from build123d import *

# Parameters (mm, degrees)
SKETCH2_W           = 60
SKETCH2_H           = 10
SKETCH2_W_2         = 11.850089675
SKETCH2_H_2         = 89.916
SKETCH2_R           = 4
SKETCH2_W_3         = 10.16
SKETCH2_H_3         = 76.2
SKETCH2_R_2         = 3.175
SKETCH2_R_3         = 4.7625
SKETCH2_H_4         = 63.685061478
SKETCH2_H_5         = 63.685061479
BOSS_EXTRUDE1_DEPTH = 10


with BuildPart() as part:
    # Sketch2 → Boss-Extrude1 (new body)
    with BuildSketch(Plane.XY):
        with BuildLine():
            Line((-102.394461083, 316.728644457), (-121.859662508, 219.58578935))
            Line((-121.859662508, 219.58578935), (-459.721789204, 219.58578935))
            Line((-459.721789204, 219.58578935), (-459.721789204, -230.782639429))
            ThreePointArc((-459.721789204, -230.782639429), (-437.403325931, -284.664176156), (-383.521789204, -306.982639429))
            Line((-383.521789204, -306.982639429), (-252, -306.982639429))
            Line((-252, -306.982639429), (-252, -317.142639429))
            Line((-252, -317.142639429), (-55.8292, -317.142639429))
            Line((-55.8292, -317.142639429), (-55.8292, -306.982639429))
            Line((-55.8292, -306.982639429), (55.8292, -306.982639429))
            Line((55.8292, -306.982639429), (55.8292, -317.142639429))
            Line((55.8292, -317.142639429), (252, -317.142639429))
            Line((252, -317.142639429), (252, -306.982639429))
            Line((252, -306.982639429), (383.521789204, -306.982639429))
            ThreePointArc((383.521789204, -306.982639429), (437.403325931, -284.664176156), (459.721789204, -230.782639429))
            Line((459.721789204, -230.782639429), (459.721789204, 152.75736057))
            Line((459.721789204, 152.75736057), (408.921789204, 152.75736057))
            Line((408.921789204, 152.75736057), (411.84465756, 142.597360571))
            Line((411.84465756, 142.597360571), (335.64465756, 142.597360571))
            Line((335.64465756, 142.597360571), (335.022501884, 152.75736057))
            Line((335.022501884, 152.75736057), (135.250547773, 152.75736057))
            Line((135.250547773, 152.75736057), (102.394461083, 316.728644457))
            Line((102.394461083, 316.728644457), (-102.394461083, 316.728644457))
        make_face()
        with Locations((-365.16, -186.254154613)):
            Rectangle(SKETCH2_W, SKETCH2_H, mode=Mode.SUBTRACT)
        with Locations((-311.557332494, -172.10863943)):
            Rectangle(SKETCH2_W_2, SKETCH2_H_2, mode=Mode.SUBTRACT)
        with Locations((-240.16, -186.254154613)):
            Rectangle(SKETCH2_W, SKETCH2_H, mode=Mode.SUBTRACT)
        with Locations((-172.69, -269.442639429)):
            Circle(SKETCH2_R, mode=Mode.SUBTRACT)
        with Locations((-205.08, -256.782661115)):
            Rectangle(SKETCH2_W_3, SKETCH2_H_3, mode=Mode.SUBTRACT)
        with Locations((-172.69, -239.442639429)):
            Circle(SKETCH2_R, mode=Mode.SUBTRACT)
        with Locations((-117.38, -269.442639429)):
            Circle(SKETCH2_R, mode=Mode.SUBTRACT)
        with Locations((-117.38, -239.442639429)):
            Circle(SKETCH2_R, mode=Mode.SUBTRACT)
        with Locations((-84.92, -256.782661115)):
            Rectangle(SKETCH2_W_3, SKETCH2_H_3, mode=Mode.SUBTRACT)
        with BuildLine():
            ThreePointArc((-108.5, -194.170881029), (-95, -207.670881029), (-108.5, -221.170881029))
            Line((-108.5, -221.170881029), (-138.5, -221.170881029))
            ThreePointArc((-138.5, -221.170881029), (-152, -207.670881029), (-138.5, -194.170881029))
            Line((-138.5, -194.170881029), (-108.5, -194.170881029))
        make_face(mode=Mode.SUBTRACT)
        with Locations((-336.55027219, -94.687385458)):
            Circle(SKETCH2_R_2, mode=Mode.SUBTRACT)
        with Locations((-378.573819589, -5.78737531)):
            Circle(SKETCH2_R_2, mode=Mode.SUBTRACT)
        with Locations((-365.16, -74.446988355)):
            Rectangle(SKETCH2_W, SKETCH2_H, mode=Mode.SUBTRACT)
        Polygon((-270.16, -69.446988355), (-210.16, -69.446988355), (-210.16, -8.96237531), (-200, -8.96237531), (-200, -85.16237531), (-210.16, -85.16237531), (-210.16, -79.446988355), (-270.16, -79.446988355), align=None, mode=Mode.SUBTRACT)
        with Locations((-336.55027219, -5.787385458)):
            Circle(SKETCH2_R_2, mode=Mode.SUBTRACT)
        with Locations((-84.92, -47.06237531)):
            Rectangle(SKETCH2_W_3, SKETCH2_H_3, mode=Mode.SUBTRACT)
        with Locations((0, -78.38263943)):
            Circle(SKETCH2_R_2, mode=Mode.SUBTRACT)
        with Locations((311.557332494, -172.10863943)):
            Rectangle(SKETCH2_W_2, SKETCH2_H_2, mode=Mode.SUBTRACT)
        with Locations((95.25, -84.73263943)):
            Circle(SKETCH2_R_3, mode=Mode.SUBTRACT)
        with Locations((195.58, -147.752560311)):
            Rectangle(SKETCH2_W_3, SKETCH2_H_4, mode=Mode.SUBTRACT)
        with Locations((195.58, -20.382437355)):
            Rectangle(SKETCH2_W_3, SKETCH2_H_5, mode=Mode.SUBTRACT)
        with Locations((336.550272189, -94.687385458)):
            Circle(SKETCH2_R_2, mode=Mode.SUBTRACT)
        with Locations((336.550272189, -5.787385458)):
            Circle(SKETCH2_R_2, mode=Mode.SUBTRACT)
        with Locations((378.573819589, -5.78737531)):
            Circle(SKETCH2_R_2, mode=Mode.SUBTRACT)
        with Locations((-311.557332494, 7.72336057)):
            Rectangle(SKETCH2_W_2, SKETCH2_H_2, mode=Mode.SUBTRACT)
        with Locations((-412.75027219, 83.112614542)):
            Circle(SKETCH2_R_2, mode=Mode.SUBTRACT)
        with Locations((-336.55027219, 83.112614542)):
            Circle(SKETCH2_R_2, mode=Mode.SUBTRACT)
        with Locations((-172.2755, 25.75736057)):
            Circle(SKETCH2_R_3, mode=Mode.SUBTRACT)
        with Locations((-81.7245, 25.75736057)):
            Circle(SKETCH2_R_3, mode=Mode.SUBTRACT)
        with Locations((-172.2755, 127.35736057)):
            Circle(SKETCH2_R_3, mode=Mode.SUBTRACT)
        with Locations((-81.7245, 127.35736057)):
            Circle(SKETCH2_R_3, mode=Mode.SUBTRACT)
        with Locations((81.7245, 25.75736057)):
            Circle(SKETCH2_R_3, mode=Mode.SUBTRACT)
        with Locations((172.2755, 25.75736057)):
            Circle(SKETCH2_R_3, mode=Mode.SUBTRACT)
        with Locations((81.7245, 127.35736057)):
            Circle(SKETCH2_R_3, mode=Mode.SUBTRACT)
        with Locations((195.58, 106.97026018)):
            Rectangle(SKETCH2_W_3, SKETCH2_H_5, mode=Mode.SUBTRACT)
        with Locations((172.2755, 127.35736057)):
            Circle(SKETCH2_R_3, mode=Mode.SUBTRACT)
        with Locations((311.557332494, 7.72336057)):
            Rectangle(SKETCH2_W_2, SKETCH2_H_2, mode=Mode.SUBTRACT)
        with Locations((336.550272189, 83.112614542)):
            Circle(SKETCH2_R_2, mode=Mode.SUBTRACT)
        with Locations((412.750272189, 83.112614542)):
            Circle(SKETCH2_R_2, mode=Mode.SUBTRACT)
        with Locations((-339.071789204, 206.88578935)):
            Circle(SKETCH2_R, mode=Mode.SUBTRACT)
        with Locations((-288.271789204, 206.88578935)):
            Circle(SKETCH2_R, mode=Mode.SUBTRACT)
        with Locations((-440.671789204, 206.88578935)):
            Circle(SKETCH2_R, mode=Mode.SUBTRACT)
        with Locations((-389.871789204, 206.88578935)):
            Circle(SKETCH2_R, mode=Mode.SUBTRACT)
    extrude(amount=-BOSS_EXTRUDE1_DEPTH)


solid = part.part
Model file for the job. Use its own axes, mm. Round coordinates to 2 decimals unless told otherwise and drop trailing zeros. Order: outer loops, then holes, each group sorted by start corner. A loop starts at its lowest first (then second) coordinate and runs counter-clockwise, first axis right, second up.
(1) Band-saw the part on C-C (x = 215). List the corners of the cut face in (y, z), then the cut area to 3 significant figures.
(2) Drill centre lines: line 1 (X direction, y = -170, z = -5); line 2 (Y direction, x = 82, z = -3.75); line 3 (X direction, y = 36, z = -9.5). Where is each one in solid material? Low to high.
(3) Pull direction Z, two halves, no side cores. Call faces 1 (the face through (-437.99, -284.07, -4.93)), 2 (the face through (-6, 4, 0)), 3 (the face through (-6, 4, -10)): released by +Z, released by -Z, zero draft, split by the parting line, or undercut.
(4) Pin check, flat tips, straight feed: pin 1 (5 mm diameter, centred on x = 412.75, y = 83.11, fed in from -Z); pin 2 (5 mm diameter, centred on y = -266.5, z = -3, fed in from +X). Stop position of each tip, or through.
(5) Band-saw the part on A-A (y = -157). List the corners of the cut face in (x, z).
(6) Band-saw the part on D-D (y = 167.5). List the corners of the cut face in (x, z), then the cut area to 3 significant figures.
(7) Band-saw the part on B-B (z = -3). Give the number of separate pieces and of enclosed holes in the cut face, then the cut area to 3 significant figures.
Verdict:
1. outline: (-317.14, -10) - (152.76, -10) - (152.76, 0) - (-317.14, 0) - close
1. area: 4,700 mm2
2. line 1: x = -459.72 to -317.48, -305.63 to 190.5, 200.66 to 305.63, 317.48 to 459.72
2. line 2: y = -317.14 to 21, 30.51 to 122.6, 132.11 to 316.73
2. line 3: x = -459.72 to -317.48, -305.63 to 305.63, 317.48 to 459.72
3. face 1: zero draft
3. face 2: released by +Z
3. face 3: released by -Z
4. pin 1: passes through
4. pin 2: stops at x = 452.1
5. outline: (-459.72, -10) - (-317.48, -10) - (-317.48, 0) - (-459.72, 0) - close; (-305.63, -10) - (190.5, -10) - (190.5, 0) - (-305.63, 0) - close; (200.66, -10) - (305.63, -10) - (305.63, 0) - (200.66, 0) - close; (317.48, -10) - (459.72, -10) - (459.72, 0) - (317.48, 0) - close
6. outline: (-459.72, -10) - (132.3, -10) - (132.3, 0) - (-459.72, 0) - close
6. area: 5,920 mm2
7. separate pieces: 1
7. enclosed holes: 43
7. area: 470,000 mm2
